```python
from build123d import *

# Parameters (mm, degrees)
SKETCH1_W           = 18
SKETCH1_H           = 11
BOSS_EXTRUDE1_DEPTH = 65
SKETCH2_W           = 18
SKETCH2_H           = 15
BOSS_EXTRUDE2_DEPTH = 5
CUT_EXTRUDE1_DEPTH  = 69.258699079


with BuildPart() as part:
    # Sketch1 → Boss-Extrude1 (new body)
    with BuildSketch(Plane.XY):
        Rectangle(SKETCH1_W, SKETCH1_H)
    extrude(amount=-BOSS_EXTRUDE1_DEPTH)

    # Sketch2 → Boss-Extrude2 (add)
    with BuildSketch(Plane(origin=(0, 5.5, 0), x_dir=(1, 0, 0), z_dir=(0, 1, 0))):
        with Locations((0, 7.5)):
            Rectangle(SKETCH2_W, SKETCH2_H)
    extrude(amount=BOSS_EXTRUDE2_DEPTH)

    # Sketch3 → Cut-Extrude1 (cut, through all)
    with BuildSketch(Plane(origin=(9, 0, 0), x_dir=(0, 0, -1), z_dir=(1, 0, 0))):
        Polygon((7.5, 10.5), (0, 3), (0, 10.5), align=None)
    extrude(amount=-CUT_EXTRUDE1_DEPTH, mode=Mode.SUBTRACT)


solid = part.part
```
Could you check a few things on this model? Use its own coordinates, in mm. A direction names the side the tool comes from. Coordinates: 2 decimals unless noted, no trailing zeros. Write each loop counter-clockwise with the first axis right and the second up, starting at its lowest first coordinate (ties: lowest second). Pieces come first, ordered by that corner, then holes. Notation, with made-up numbers: (42, -7.5) -> (95, -7.5) arc R30 ccw to (95, 14.5) -> close; hole circle Ø1 at (-9, 28). An arc over 180 degrees is marked (long way). Write item = value, one per line. Start each with the question number.
(1) I want a section at B-B (y = 6.25). Please give me the cut outline in (x, z), plus the area to 4 significant figures.
(2) I want a section at C-C (z = -57). Please give me the cut outline in (x, y), plus the area to 3 significant figures.
(3) I need wall thicknesses on line 1 (Y direction, x = -1.75, z = -48); line 2 (Z direction, x = 3.75, y = 9.75); line 3 (Z direction, x = 6, y = 4.75). Which ranges of each line are inside material? Lowest first, please. Write a range as [from, to].
(4) Will this pin go through, and if not, where does the flat tip stop? pin 1 (5.5 mm diameter, centred on x = -1.5, z = -32, fed in from +Y).
(5) I want a section at A-A (x = -6.75). Please give me the cut outline in (y, z), plus the area to 3 significant figures.
(6) Which directions (+Z, -Z, +X, -X, +Y, -Y) give clear straight access to the entire face, cutting with the end or side of a thin tool? Please do faces 1 (the face through (9, 1, -32)), 2 (the face through (0, 8, -15)).
Result set:
q1.outline = (-9, -15) -> (9, -15) -> (9, -3.25) -> (-9, -3.25) -> close
q1.area = 211.5 mm2
q2.outline = (-9, -5.5) -> (9, -5.5) -> (9, 5.5) -> (-9, 5.5) -> close
q2.area = 198 mm2
q3.line_1 = [-5.5, 5.5]
q3.line_2 = [-15, -6.75]
q3.line_3 = [-65, -1.75]
q4.pin_1 = 5.5
q5.outline = (-5.5, -65) -> (5.5, -65) -> (5.5, -15) -> (10.5, -15) -> (10.5, -7.5) -> (3, 0) -> (-5.5, 0) -> close
q5.area = 762 mm2
q6.face_1 = +Z, -Z, +X, +Y, -Y
q6.face_2 = -Z, +X, -X, +Y
